```python
from build123d import *

# Parameters (mm, degrees)
SKETCH1_W           = 200
SKETCH1_H           = 134
BOSS_EXTRUDE1_DEPTH = 2
SKETCH2_R           = 0.5
CUT_EXTRUDE1_DEPTH  = 211.933638854
SKETCH3_W           = 200
SKETCH3_H           = 2
BOSS_EXTRUDE2_DEPTH = 5


with BuildPart() as part:
    # Sketch1 → Boss-Extrude1 (new body)
    with BuildSketch(Plane(origin=(0, 0, 0), x_dir=(1, 0, 0), z_dir=(0, 1, 0))):
        Rectangle(SKETCH1_W, SKETCH1_H)
    extrude(amount=BOSS_EXTRUDE1_DEPTH)

    # Sketch2 → Cut-Extrude1 (cut, through all)
    with BuildSketch(Plane(origin=(100, 0, 0), x_dir=(0, 0, -1), z_dir=(1, 0, 0))):
        with Locations((-66, 1)):
            Circle(SKETCH2_R)
    extrude(amount=-CUT_EXTRUDE1_DEPTH, mode=Mode.SUBTRACT)

    # Sketch3 → Boss-Extrude2 (add)
    with BuildSketch(Plane.XY.offset(67)):
        with Locations((0, 1)):
            Rectangle(SKETCH3_W, SKETCH3_H)
    extrude(amount=BOSS_EXTRUDE2_DEPTH)


solid = part.part
```
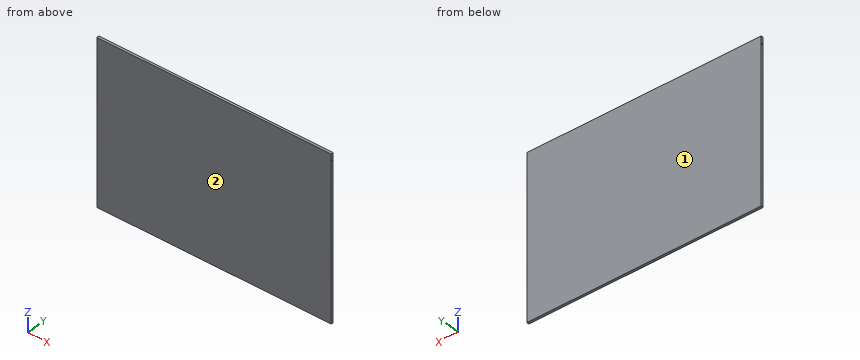
Part model, mm, in its own coordinate system. Face numbers are marked on the shaded views. Round coordinates to 2 decimals unless told otherwise and drop trailing zeros. Answer in a Markdown table with one row per item. Add a question column.
Q1. Mould opens along Y. For the marked faces 1 and 2 say: +Y half, -Y half, draft (parallel to the pull), parting line (faces both ways), or undercut.
Q2. Wall check: L1, parallel to Y at x = -57, z = 66; L2, parallel to Z at x = 1.5, y = 0.85; L3, parallel to Z at x = -80, y = 0.6. Give the ranges that are in metal, low to high. Write a range as from..to.
Q3. Pin check, flat tip, straight feed: pin 1 (10 mm diameter, centred on x = 72.5, z = 43, fed in from -Y). Stop position of the tip, or through.
Established:
| question | item | result |
|---|---|---|
| 1 | face 1 | +Y half |
| 1 | face 2 | -Y half |
| 2 | L1 | y = 0..0.5, 1.5..2 |
| 2 | L2 | z = -67..65.52, 66.48..72 |
| 2 | L3 | z = -67..65.7, 66.3..72 |
| 3 | pin 1 | stops at y = 0 |
